```python
from build123d import *

# Parameters (mm, degrees)
F0_R     = 6
F0_R_2   = 2.5
F1_DEPTH = 3
F2_DEPTH = 6
F3_SIZE  = 1


with BuildPart() as f1:
    # F0 (on Top) → F1 (new body)
    with BuildSketch(Plane.XY):
        Circle(F0_R)
        Circle(F0_R_2, mode=Mode.SUBTRACT)
        Circle(F0_R_2)
    extrude(amount=-F1_DEPTH)

    # F0 (on Top) → F2 (join)
    with BuildSketch(Plane.XY):
        Circle(F0_R_2)
    extrude(amount=F2_DEPTH)

    # F3
    f3_edges = [f1.edges().sort_by_distance(p)[0] for p in [
        (-2.5, 0, 6),
        (-6, 0, -3),
    ]]
    chamfer(f3_edges, length=F3_SIZE)


solid = f1.part
```
Input: part model. Units: mm. Frame: model coordinates. A direction names the side the tool comes from. Give positions to 0.01 mm unless a question says otherwise; leave off trailing zeros. Loops run counter-clockwise (first coordinate to the right, second up) from the corner with the lowest first, then second, coordinate; pieces in that order, holes last. Notation, with made-up numbers: M 52.25,19 L 97.25,19 A23 ccw 97.25,41 Z; hole C -25,58 d9. An arc over 180 degrees is marked long. Answer as CSV lines item,"result". Start each with the question number.
1. Section A-A on x = 0. Return loops of the section in (y, z), plus the area to 3 significant figures.
2. Pin query (flat end, axial travel): P1, Ø4, axis at x = 3, z = 3, coming from the -Y side; P2, Ø3, axis at y = -2.5, z = 0.5, coming from the +X side. Return the tip coordinate at first contact, or that it passes through.
3. Reachability of faces 1 (the face through (-0.54, -2.44, 2.46)), 2 (the face through (0, 0, 6)) from +Z, -Z, +X, -X, +Y, -Y: full face, straight path, thin tool, end or side. Return the list, or none.
4. Line query: L1, parallel to Z at x = 3.5, y = 2.25; L2, parallel to Y at x = -2, z = 1.5; L3, parallel to Z at x = 2, y = -5.5. Output: solid intervals per line, ascending.
5. Section C-C on z = 3.5. Return loops of the section in (x, y), plus the area to 3 significant figures.
Computed values:
1,outline,"M -6,-2 L -5,-3 L 5,-3 L 6,-2 L 6,0 L 2.5,0 L 2.5,5 L 1.5,6 L -1.5,6 L -2.5,5 L -2.5,0 L -6,0 Z"
1,area,"64.0 mm²"
2,P1,"stops at y = -2.29"
2,P2,"stops at x = 5.9"
3,face 1,"+Z"
3,face 2,"+Z, +X, -X, +Y, -Y"
4,L1,"z = -3 to 0"
4,L2,"y = -1.5 to 1.5"
4,L3,"z = -2.15 to 0"
5,outline,"C 0,0 d5"
5,area,"19.6 mm²"
